from build123d import *

# Parameters (mm, degrees)
SKETCH1_R           = 2.75
BOSS_EXTRUDE1_DEPTH = 11
CUT_EXTRUDE1_DEPTH  = 23.341105613
BOSS_EXTRUDE2_START = 9
BOSS_EXTRUDE2_DEPTH = 10
CUT_EXTRUDE2_START  = -13
CUT_EXTRUDE2_DEPTH  = 21
BOSS_EXTRUDE3_DEPTH = 5


with BuildPart() as part:
    # Sketch1 → Boss-Extrude1 (new, symmetric)
    with BuildSketch(Plane(origin=(0, 0, 0), x_dir=(0, 0, -1), z_dir=(1, 0, 0))):
        Circle(SKETCH1_R)
    extrude(amount=BOSS_EXTRUDE1_DEPTH, both=True)

    # Sketch2 → Cut-Extrude1 (cut, through all)
    with BuildSketch(Plane(origin=(11, 0, 0), x_dir=(0, 0, -1), z_dir=(1, 0, 0))):
        with BuildLine():
            Line((-1.85, 2.034698995), (-1.85, -2.034698995))
            ThreePointArc((-1.85, -2.034698995), (-2.75, 0), (-1.85, 2.034698995))
        make_face()
        with BuildLine():
            Line((1.85, 2.034698995), (1.85, -2.034698995))
            ThreePointArc((1.85, -2.034698995), (2.75, 0), (1.85, 2.034698995))
        make_face()
    extrude(amount=-CUT_EXTRUDE1_DEPTH, mode=Mode.SUBTRACT)

    # Sketch3 → Boss-Extrude2 (add)
    with BuildSketch(Plane(origin=(11, 0, 0), x_dir=(0, 0, -1), z_dir=(1, 0, 0)).offset(BOSS_EXTRUDE2_START)):
        with BuildLine():
            Line((-3.85, 2.782085549), (-3.85, -2.782085549))
            ThreePointArc((-3.85, -2.782085549), (0, -4.75), (3.85, -2.782085549))
            Line((3.85, -2.782085549), (3.85, 2.782085549))
            ThreePointArc((3.85, 2.782085549), (0, 4.75), (-3.85, 2.782085549))
        make_face()
        with BuildLine():
            Line((-1.85, 2.034698995), (-1.85, -2.034698995))
            ThreePointArc((-1.85, -2.034698995), (0, -2.75), (1.85, -2.034698995))
            Line((1.85, -2.034698995), (1.85, 2.034698995))
            ThreePointArc((1.85, 2.034698995), (0, 2.75), (-1.85, 2.034698995))
        make_face(mode=Mode.SUBTRACT)
    extrude(amount=-BOSS_EXTRUDE2_DEPTH)

    # Sketch5 → Cut-Extrude2 (cut)
    with BuildSketch(Plane.ZY.offset(3).offset(CUT_EXTRUDE2_START)):
        with BuildLine():
            Line((1.85, -2.034698995), (1.85, 2.034698995))
            ThreePointArc((1.85, 2.034698995), (0, 2.75), (-1.85, 2.034698995))
            Line((-1.85, 2.034698995), (-1.85, -2.034698995))
            ThreePointArc((-1.85, -2.034698995), (0, -2.75), (1.85, -2.034698995))
        make_face()
    extrude(amount=CUT_EXTRUDE2_DEPTH, mode=Mode.SUBTRACT)

    # Sketch6 → Boss-Extrude3 (add)
    with BuildSketch(Plane.ZY.offset(-10)):
        with BuildLine():
            ThreePointArc((3.85, 2.782085549), (0, 4.75), (-3.85, 2.782085549))
            Line((-3.85, 2.782085549), (-3.85, -2.782085549))
            ThreePointArc((-3.85, -2.782085549), (0, -4.75), (3.85, -2.782085549))
            Line((3.85, -2.782085549), (3.85, 2.782085549))
        make_face()
        with BuildLine():
            Line((-1.4, -2.877498914), (-1.4, 2.877498914))
            ThreePointArc((-1.4, 2.877498914), (3.2, 0), (-1.4, -2.877498914))
        make_face(mode=Mode.SUBTRACT)
    extrude(amount=BOSS_EXTRUDE3_DEPTH)


solid = part.part
CAD build for the part. Positions are in the model's coordinates, mm. A direction names the side the tool comes from. Coordinates: 2 decimals unless noted, no trailing zeros. Write each loop counter-clockwise with the first axis right and the second up, starting at its lowest first coordinate (ties: lowest second). Pieces come first, ordered by that corner, then holes. Notation, with made-up numbers: M 32,73.5 L 67,73.5 A21 ccw 67,105.5 Z; hole C 74.25,-26 d10. An arc over 180 degrees is marked long. Answer as a JSON object with one key per item and string values. Group by question number.
1) Saw through at A-A (x = 17.5). Write the cut outline in (y, z).
2) Tool access for faces 4 (the face through (5, 0, -2)), 5 (the face through (8, 0, -1.4)), 6 (the face through (16, 0, -1.85)): list every direction of +Z, -Z, +X, -X, +Y, -Y with a clear straight run to the whole face (end or side of a thin tool).
3) Saw through at C-C (y = 0). Write the cut outline in (x, z).
4) Wall check: line 1 (Z direction, x = 8.45, y = 0); line 2 (Y direction, x = 16, z = 0); line 3 (Y direction, x = 8.7, z = 0). Give the ranges that are in metal, low to high. Write a range as from..to.
5) Mould opens along Y. For faces 1 (the face through (12.6, 4.75, 0.06)), 2 (the face through (15.56, -2.75, 0.03)), 3 (the face through (20, 0, 3)) say: +Y half, -Y half, draft (parallel to the pull), parting line (faces both ways), or undercut.
6) Pin check, flat tip, straight feed: pin 1 Ø1.5 at (x, z) = (8, 1.5) entering from -Y. Stop position of the tip, or through.
7) Saw through at D-D (x = 8.75). Write the cut outline in (y, z), plus the area to 3 significant figures.
8) Saw through at B-B (z = 0). Write the cut outline in (x, y), plus the area to 3 significant figures.
Values follow:
{
 "1": {"outline": "M -2.78,-3.85 L 2.78,-3.85 A4.75 ccw 2.78,3.85 L -2.78,3.85 A4.75 ccw Z; hole M -2.03,-1.85 L 2.03,-1.85 A2.75 ccw 2.03,1.85 L -2.03,1.85 A2.75 ccw Z"},
 "2": {"face 4": "+Z, -Z, -X, +Y, -Y", "face 5": "-X", "face 6": "+X"},
 "3": {"outline": "M 5,-3.85 L 20,-3.85 L 20,-1.85 L 11,-1.85 L 11,1.85 L 20,1.85 L 20,3.85 L 5,3.85 L 5,3.2 L 10,3.2 L 10,-1.4 L 5,-1.4 Z"},
 "4": {"line 1": "z = -3.85..-1.4, 3.2..3.85", "line 2": "y = -4.75..-2.75, 2.75..4.75", "line 3": "y = -4.75..-3.2, 3.2..4.75"},
 "5": {"face 1": "+Y half", "face 2": "undercut", "face 3": "draft"},
 "6": {"pin 1": "stops at y = -4.69"},
 "7": {"outline": "M -2.78,-3.85 L 2.78,-3.85 A4.75 ccw 2.78,3.85 L -2.78,3.85 A4.75 ccw Z; hole M -2.88,-1.4 L 2.88,-1.4 A3.2 ccw long Z", "area": "39.3 mm2"},
 "8": {"outline": "M 5,-4.75 L 20,-4.75 L 20,-2.75 L 11,-2.75 L 11,2.75 L 20,2.75 L 20,4.75 L 5,4.75 L 5,3.2 L 10,3.2 L 10,-3.2 L 5,-3.2 Z", "area": "61.0 mm2"}
}
